```python
from build123d import *

# Parameters (mm, degrees)
BOSS_EXTRUDE1_DEPTH = 10
CHAMFER1_SIZE       = 7.802060087
CHAMFER1_SIZE_2     = 10
BOSS_EXTRUDE2_DEPTH = 20
SKETCH7_R           = 1.5
CUT_EXTRUDE1_DEPTH  = 20
CUT_EXTRUDE3_DEPTH  = 20
FILLET5_R           = 20
FILLET6_R           = 10
SKETCH10_W          = 5.3
SKETCH10_H          = 4.24
CUT_EXTRUDE4_DEPTH  = 273.805653344
SKETCH11_W          = 3.75
SKETCH11_H          = 144.691495626
CUT_EXTRUDE5_DEPTH  = 370.011076387
BOSS_EXTRUDE4_DEPTH = 12.5
SKETCH12_W          = 2
SKETCH12_H          = 1.5
CUT_EXTRUDE6_DEPTH  = 144.691496


with BuildPart() as part:
    # Sketch2 → Boss-Extrude1 (new, symmetric)
    with BuildSketch(Plane(origin=(0, 0, 0), x_dir=(0, 0, -1), z_dir=(1, 0, 0))):
        Polygon((36.072931518, 122.5), (-51.279924706, -117.5), (-51.279924706, -192), (-46.279924706, -192), (-46.279924706, -151.5), (-39.679924706, -151.5), (-39.679924706, -192), (-35.679924706, -192), (-35.679924706, -117.5), (-42.766502526, -117.5), (42.766502526, 117.5), (192.766502526, 117.5), (192.766502526, 122.5), align=None)
    extrude(amount=BOSS_EXTRUDE1_DEPTH, both=True)

    # Chamfer1
    # the kernel refuses this chamfer: 10, 7.802060087 mm, written as the material it adds along each edge
    with BuildSketch(Plane(origin=(-10, -117.5, 42.766502526), x_dir=(0, 0.9542611885293297, -0.298974219735734), z_dir=(1, 0, 0))) as chamfer1_piece_1_section:
        Polygon((CHAMFER1_SIZE * 0.998967402661, -CHAMFER1_SIZE * 0.0454326803806), (CHAMFER1_SIZE_2 * 0.298974219736, -CHAMFER1_SIZE_2 * 0.954261188529), (0, 0), align=None)
    chamfer1_piece_1 = extrude(amount=20, mode=Mode.PRIVATE)
    chamfer1_piece_1 = split(chamfer1_piece_1, bisect_by=Plane(origin=(0, -114.855220314, 35.679924706), z_dir=(0, 0, 1)), keep=Keep.TOP, mode=Mode.PRIVATE)
    add(chamfer1_piece_1)

    # Sketch6 → Boss-Extrude2 (add)
    with BuildSketch(Plane(origin=(10, 0, 0), x_dir=(0, 0, -1), z_dir=(1, 0, 0))):
        Polygon((-51.279924706, -180), (-66.279924706, -192), (-51.279924706, -192), align=None)
        Polygon((-35.679924706, -192), (-20.679924706, -192), (-35.679924706, -180), align=None)
    extrude(amount=-BOSS_EXTRUDE2_DEPTH)

    # Sketch7 → Cut-Extrude1 (cut)
    with BuildSketch(Plane(origin=(0, -192, 0), x_dir=(-1, 0, 0), z_dir=(0, -1, 0))):
        with Locations(Location((0, -56.279924706, 0), (0, 0, 90))):
            Circle(SKETCH7_R)
        with Locations(Location((0, -30.179924706, 0), (0, 0, 90))):
            Circle(SKETCH7_R)
    extrude(amount=-CUT_EXTRUDE1_DEPTH, mode=Mode.SUBTRACT)

    # Sketch9 → Cut-Extrude3 (cut)
    with BuildSketch(Plane(origin=(0, -187, 0), x_dir=(-1, 0, 0), z_dir=(0, -1, 0))):
        Polygon((2.75, -57.867637946), (2.75, -54.692211466), (0, -53.104498226), (-2.75, -54.692211466), (-2.75, -57.867637946), (0, -59.455351187), align=None)
        Polygon((2.75, -31.767637946), (2.75, -28.592211466), (0, -27.004498226), (-2.75, -28.592211466), (-2.75, -31.767637946), (0, -33.355351187), align=None)
    extrude(amount=-CUT_EXTRUDE3_DEPTH, mode=Mode.SUBTRACT)

    # Fillet5
    fillet5_edges = [part.edges().sort_by_distance(p)[0] for p in [
        (0, -117.5, 51.279924706),
    ]]
    fillet(fillet5_edges, radius=FILLET5_R)

    # Fillet6
    fillet6_edges = [part.edges().sort_by_distance(p)[0] for p in [
        (0, 122.5, -36.072931518),
    ]]
    fillet(fillet6_edges, radius=FILLET6_R)

    # Sketch10 → Cut-Extrude4 (cut, through all)
    with BuildSketch(Plane(origin=(10, 0, 0), x_dir=(0, 0, -1), z_dir=(1, 0, 0))):
        with Locations((-63.629924706, -189.88)):
            Rectangle(SKETCH10_W, SKETCH10_H)
        with Locations((-23.329924706, -189.88)):
            Rectangle(SKETCH10_W, SKETCH10_H)
    extrude(amount=-CUT_EXTRUDE4_DEPTH, mode=Mode.SUBTRACT)

    # Sketch11 → Cut-Extrude5 (cut, through all)
    with BuildSketch(Plane(origin=(0, 122.5, 0), x_dir=(1, 0, 0), z_dir=(0, 1, 0))):
        with Locations((-8.125, 120.420754713)):
            Rectangle(SKETCH11_W, SKETCH11_H)
        with Locations((8.125, 120.420754713)):
            Rectangle(SKETCH11_W, SKETCH11_H)
    extrude(amount=-CUT_EXTRUDE5_DEPTH, mode=Mode.SUBTRACT)

    # Sketch13 → Boss-Extrude4 (add)
    with BuildSketch(Plane(origin=(6.25, 0, 0), x_dir=(0, 0, -1), z_dir=(1, 0, 0))):
        Polygon((52.766502526, 117.5), (37.766502526, 103.762612903), (42.766502526, 117.5), align=None)
    extrude(amount=-BOSS_EXTRUDE4_DEPTH)

    # Sketch12 → Cut-Extrude6 (cut)
    with BuildSketch(Plane(origin=(0, 0, -192.766502526), x_dir=(-1, 0, 0), z_dir=(0, 0, -1))):
        with Locations((-5.25, 120)):
            Rectangle(SKETCH12_W, SKETCH12_H)
        with Locations((5.25, 120)):
            Rectangle(SKETCH12_W, SKETCH12_H)
    extrude(amount=-CUT_EXTRUDE6_DEPTH, mode=Mode.SUBTRACT)


solid = part.part
```
For this review, take the finished solid that the model builds, in its own axes (mm). A direction names the side the tool comes from. Round coordinates to 2 decimals unless told otherwise and drop trailing zeros. Order: outer loops, then holes, each group sorted by start corner. A loop starts at its lowest first (then second) coordinate and runs counter-clockwise, first axis right, second up. Notation, with made-up numbers: (-20, 79.25) -> (34, 79.25) arc R15 ccw to (34, 83.25) -> close; hole circle Ø7 at (-13, -23). An arc over 180 degrees is marked (long way). Use a Markdown table: item, result.
Item 1: Take a section at A-A (z = -105). State the section outline as (x, y) points, plus the area to 3 significant figures.
Resolved:
| item | result |
|---|---|
| outline | (-6.25, 117.5) -> (6.25, 117.5) -> (6.25, 119.25) -> (4.25, 119.25) -> (4.25, 120.75) -> (6.25, 120.75) -> (6.25, 122.5) -> (-6.25, 122.5) -> (-6.25, 120.75) -> (-4.25, 120.75) -> (-4.25, 119.25) -> (-6.25, 119.25) -> close |
| area | 56.5 mm² |
Item 2: Draft analysis for pull direction Z (two halves, no side actions). For faces 6 (the flat face through (0, -172, 46.28)), 7 (the flat face through (2.362, -182.101, 53.906)), 8 (the flat face through (0, -151.5, 43)), 9 (the flat face through (2.36, -182.21, 32.92)), state which applies: +Z half, -Z half, draft (parallel to the pull), parting line (faces both ways), or undercut.
Resolved:
| item | result |
|---|---|
| face 6 | undercut |
| face 7 | +Z half |
| face 8 | undercut |
| face 9 | -Z half |
Item 3: Take a section at C-C (z = -15.5). State the section outline as (x, y) points, plus the area to 3 significant figures.
Resolved:
| item | result |
|---|---|
| outline | (-10, 42.59) -> (10, 42.59) -> (10, 65.98) -> (-10, 65.98) -> close |
| area | 468 mm² |
Item 4: Machinability: for faces 1 (the flat face through (0, -192, 54)), 2 (the flat face through (0, 117.5, -122)), 3 (the flat face through (0, -147, 35.68)), 4 (the flat face through (0, -171, 39.68)), 5 (the flat face through (0, -150, 51.28)), which of the approach directions +Z, -Z, +X, -X, +Y, -Y give a long, thin tool a straight path to every point of the face, cutting with its end or side? Answer none if there is none.
Resolved:
| item | result |
|---|---|
| face 1 | +Z, -Z, +X, -X, -Y |
| face 2 | -Z, +X, -X, -Y |
| face 3 | -Z, +X, -X |
| face 4 | +X, -X, -Y |
| face 5 | +Z, +X, -X, +Y |
Item 5: For line 1 along Y through (x, z) = (3.5, -110.5); line 2 along Z through (x, y) = (-0.5, 45.5); line 3 along Z through (x, y) = (-5, 85), list the stretches that pass through material, from the lowest coordinate up. Write a range as [from, to].
Resolved:
| item | result |
|---|---|
| line 1 | y = [117.5, 122.5] |
| line 2 | z = [-16.56, -8.05] |
| line 3 | z = [-30.94, -22.42] |
Item 6: For pin 1 (1.9 mm diameter, centred on x = 8.5, z = -46, fed in from -Y); pin 2 (3.5 mm diameter, centred on x = 0, z = 56.28, fed in from +Y); pin 3 (0.9 mm diameter, centred on y = 121.5, z = -140, fed in from +X); pin 4 (2.5 mm diameter, centred on y = -184.5, z = 30, fed in from -X), all flat-tipped, find the tip position at first contact; note any pin that passes through.
Resolved:
| item | result |
|---|---|
| pin 1 | stops at y = 117.5 |
| pin 2 | stops at y = -187 |
| pin 3 | stops at x = 6.25 |
| pin 4 | stops at x = -10 |
Item 7: Take a section at B-B (y = 81). State the section outline as (x, z) points, plus the area to 3 significant figures.
Resolved:
| item | result |
|---|---|
| outline | (-10, -29.48) -> (10, -29.48) -> (10, -20.97) -> (-10, -20.97) -> close |
| area | 170 mm² |
